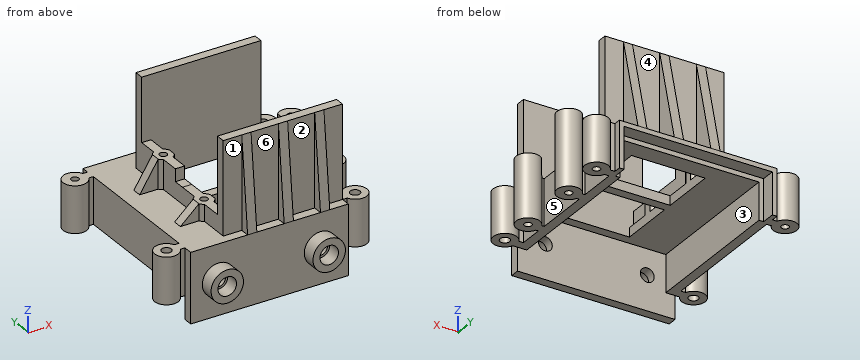
from build123d import *

# Parameters (mm, degrees)
ESQUISSE1_W              = 34
ESQUISSE1_H              = 15
BOSS_EXTRU_1_DEPTH       = 2
ESQUISSE2_R              = 1.5
ENL_V_MAT_EXTRU_1_DEPTH  = 2
BOSS_EXTRU_2_DEPTH       = 35
ENL_V_MAT_EXTRU_2_DEPTH  = 3
ESQUISSE5_R              = 3.5
ESQUISSE5_R_2            = 2
BOSS_EXTRU_3_DEPTH       = 3
ENL_V_START              = -2
ESQUISSE6_W              = 14
ESQUISSE6_H              = 12
ENL_V_MAT_EXTRU_3_DEPTH  = 2
ESQUISSE7_W              = 14
ESQUISSE7_H              = 12
ENL_V_MAT_EXTRU_4_DEPTH  = 2
ESQUISSE8_W              = 3
ESQUISSE8_H              = 12
ENL_V_MAT_EXTRU_5_DEPTH  = 2
BOSS_EXTRU_4_START       = -2
ESQUISSE9_W              = 1.1
ESQUISSE9_H              = 12
BOSS_EXTRU_4_DEPTH       = 2
ESQUISSE10_R             = 0.8
BOSS_EXTRU_5_DEPTH       = 6.285817
ESQUISSE11_R             = 0.8
BOSS_EXTRU_6_DEPTH       = 3.585817
ESQUISSE21_W             = 4
ESQUISSE21_H             = 2
BOSS_EXTRU_12_DEPTH      = 6.285817
ENL_V_MAT_EXTRU_9_DEPTH  = 2
ESQUISSE23_W             = 4
ESQUISSE23_H             = 2
BOSS_EXTRU_13_DEPTH      = 3.585817
ENL_V_MAT_EXTRU_10_DEPTH = 2
ESQUISSE25_W             = 2
ESQUISSE25_H             = 4.092832792
ESQUISSE25_H_2           = 4.443065592
BOSS_EXTRU_14_DEPTH      = 3.585817
ESQUISSE27_W             = 2
ESQUISSE27_H             = 4.092832792
ESQUISSE27_H_2           = 4
BOSS_EXTRU_15_DEPTH      = 6.285817
BOSS_EXTRU_17_START      = -10
ESQUISSE31_R             = 1.05
BOSS_EXTRU_17_DEPTH      = 10
BOSS_EXTRU_18_START      = -10
ESQUISSE33_R             = 0.8
BOSS_EXTRU_18_DEPTH      = 10
ESQUISSE34_R             = 0.8
BOSS_EXTRU_19_DEPTH      = 16.290743
ESQUISSE35_R             = 0.8
BOSS_EXTRU_20_DEPTH      = 13.590743
BOSS_EXTRU_21_DEPTH      = 20
ENL_V_START_2            = -17.727203
ENL_V_MAT_EXTRU_14_DEPTH = 17.727203
BOSS_EXTRU_23_START      = -2
ESQUISSE39_W             = 3.585817331
ESQUISSE39_H             = 2.443065592
BOSS_EXTRU_23_DEPTH      = 2
ENL_V_START_3            = -6.290743
ESQUISSE40_W             = 1.637082072
ESQUISSE40_H             = 4.811547665
ENL_V_MAT_EXTRU_15_DEPTH = 6.290743
ENL_V_START_4            = -3.590743
ESQUISSE41_W             = 1.862657742
ESQUISSE41_H             = 4.792301475
ENL_V_MAT_EXTRU_16_DEPTH = 3.590743
BOSS_EXTRU_24_DEPTH      = 20
ENL_V_MAT_EXTRU_17_DEPTH = 17.727203


with BuildPart() as part:
    # Esquisse1 → Boss.-Extru.1 (new body)
    with BuildSketch(Plane(origin=(0, 0, 0), x_dir=(1, 0, 0), z_dir=(0, 1, 0))):
        with Locations((17, 7.5)):
            Rectangle(ESQUISSE1_W, ESQUISSE1_H)
    extrude(amount=BOSS_EXTRU_1_DEPTH)

    # Esquisse2 → Enl_v. mat.-Extru.1 (cut)
    with BuildSketch(Plane(origin=(0, 2, 0), x_dir=(1, 0, 0), z_dir=(0, 1, 0))):
        with Locations((6, 7.5)):
            Circle(ESQUISSE2_R)
        with Locations((28, 7.5)):
            Circle(ESQUISSE2_R)
    extrude(amount=-ENL_V_MAT_EXTRU_1_DEPTH, mode=Mode.SUBTRACT)

    # Esquisse3 → Boss.-Extru.2 (add)
    with BuildSketch(Plane(origin=(0, 2, 0), x_dir=(1, 0, 0), z_dir=(0, 1, 0))):
        Polygon((0, 10), (2, 10), (2, 2), (32, 2), (32, 10), (34, 10), (34, 0), (0, 0), align=None)
    extrude(amount=BOSS_EXTRU_2_DEPTH)

    # Esquisse4 → Enl_v. mat.-Extru.2 (cut)
    with BuildSketch(Plane(origin=(0, 37, 0), x_dir=(1, 0, 0), z_dir=(0, 1, 0))):
        Polygon((2, 10), (1, 10), (1, 1), (33, 1), (33, 10), (32, 10), (32, 2), (2, 2), align=None)
    extrude(amount=-ENL_V_MAT_EXTRU_2_DEPTH, mode=Mode.SUBTRACT)

    # Esquisse5 → Boss.-Extru.3 (add)
    with BuildSketch(Plane.XZ):
        with Locations((6, -7.5)):
            Circle(ESQUISSE5_R)
        with Locations((6, -7.5)):
            Circle(ESQUISSE5_R_2, mode=Mode.SUBTRACT)
        with Locations((28, -7.5)):
            Circle(ESQUISSE5_R)
        with Locations((28, -7.5)):
            Circle(ESQUISSE5_R_2, mode=Mode.SUBTRACT)
    extrude(amount=BOSS_EXTRU_3_DEPTH)

    # Esquisse6 → Enl_v. mat.-Extru.3 (cut)
    with BuildSketch(Plane(origin=(0, 0, -2), x_dir=(-1, 0, 0), z_dir=(0, 0, -1)).offset(ENL_V_START)):
        with Locations((-17, 24)):
            Rectangle(ESQUISSE6_W, ESQUISSE6_H)
    extrude(amount=ENL_V_MAT_EXTRU_3_DEPTH, mode=Mode.SUBTRACT)

    # Esquisse7 → Enl_v. mat.-Extru.4 (cut)
    with BuildSketch(Plane(origin=(0, 0, -2), x_dir=(-1, 0, 0), z_dir=(0, 0, -1)).offset(ENL_V_START)):
        with Locations((-17, 10)):
            Rectangle(ESQUISSE7_W, ESQUISSE7_H)
    extrude(amount=ENL_V_MAT_EXTRU_4_DEPTH, mode=Mode.SUBTRACT)

    # Esquisse8 → Enl_v. mat.-Extru.5 (cut)
    with BuildSketch(Plane.XY.offset(ENL_V_START)):
        with Locations((25.5, 10)):
            Rectangle(ESQUISSE8_W, ESQUISSE8_H)
        with Locations((25.5, 24)):
            Rectangle(ESQUISSE8_W, ESQUISSE8_H)
    extrude(amount=ENL_V_MAT_EXTRU_5_DEPTH, mode=Mode.SUBTRACT)

    # Esquisse9 → Boss.-Extru.4 (add)
    with BuildSketch(Plane.XY.offset(BOSS_EXTRU_4_START)):
        with Locations((10.55, 24)):
            Rectangle(ESQUISSE9_W, ESQUISSE9_H)
        with Locations((10.55, 10)):
            Rectangle(ESQUISSE9_W, ESQUISSE9_H)
    extrude(amount=BOSS_EXTRU_4_DEPTH)

    # Esquisse10 → Boss.-Extru.5 (add)
    with BuildSketch(Plane.XY):
        with BuildLine():
            Line((11.1, 24.988338073), (11.1, 23.361894727))
            ThreePointArc((11.1, 23.361894727), (7.27279708, 24.1751164), (11.1, 24.988338073))
        make_face()
        with Locations((9.27279708, 24.1751164)):
            Circle(ESQUISSE10_R, mode=Mode.SUBTRACT)
    extrude(amount=BOSS_EXTRU_5_DEPTH)

    # Esquisse11 → Boss.-Extru.6 (add)
    with BuildSketch(Plane.XY):
        with BuildLine():
            Line((11.1, 10.988338073), (11.1, 9.361894727))
            ThreePointArc((11.1, 9.361894727), (7.27279708, 10.1751164), (11.1, 10.988338073))
        make_face()
        with Locations((9.27279708, 10.1751164)):
            Circle(ESQUISSE11_R, mode=Mode.SUBTRACT)
    extrude(amount=BOSS_EXTRU_6_DEPTH)

    # Esquisse21 → Boss.-Extru.12 (add)
    with BuildSketch(Plane.XY):
        with Locations((5.540746272, 24.1751164)):
            Rectangle(ESQUISSE21_W, ESQUISSE21_H)
    extrude(amount=BOSS_EXTRU_12_DEPTH)

    # Esquisse22 → Enl_v. mat.-Extru.9 (cut)
    with BuildSketch(Plane(origin=(0, 25.1751164, 0), x_dir=(1, 0, 0), z_dir=(0, 1, 0))):
        Polygon((3.540746272, 0), (7.540746272, -6.285817331), (3.540746272, -6.285817331), align=None)
    extrude(amount=-ENL_V_MAT_EXTRU_9_DEPTH, mode=Mode.SUBTRACT)

    # Esquisse23 → Boss.-Extru.13 (add)
    with BuildSketch(Plane.XY):
        with Locations((5.540746272, 10.1751164)):
            Rectangle(ESQUISSE23_W, ESQUISSE23_H)
    extrude(amount=BOSS_EXTRU_13_DEPTH)

    # Esquisse24 → Enl_v. mat.-Extru.10 (cut)
    with BuildSketch(Plane.XZ.offset(-9.1751164)):
        Polygon((7.540746272, 3.585817331), (3.540746272, 0), (3.540746272, 3.585817331), align=None)
    extrude(amount=-ENL_V_MAT_EXTRU_10_DEPTH, mode=Mode.SUBTRACT)

    # Esquisse25 → Boss.-Extru.14 (add)
    with BuildSketch(Plane.XY):
        with Locations((9.27279708, 13.953583604)):
            Rectangle(ESQUISSE25_W, ESQUISSE25_H)
        with Locations((9.27279708, 6.221532796)):
            Rectangle(ESQUISSE25_W, ESQUISSE25_H_2)
    extrude(amount=BOSS_EXTRU_14_DEPTH)

    # Esquisse27 → Boss.-Extru.15 (add)
    with BuildSketch(Plane.XY):
        with Locations((9.27279708, 27.953583604)):
            Rectangle(ESQUISSE27_W, ESQUISSE27_H)
        with Locations((9.27279708, 20.443065592)):
            Rectangle(ESQUISSE27_W, ESQUISSE27_H_2)
    extrude(amount=BOSS_EXTRU_15_DEPTH)

    # Esquisse31 → Boss.-Extru.17 (add)
    with BuildSketch(Plane.XY.offset(BOSS_EXTRU_17_START)):
        with BuildLine():
            Line((-1, 4), (0, 4))
            Line((0, 4), (0, 2))
            Line((0, 2), (-1, 2))
            ThreePointArc((-1, 2), (-5.895740821, 3), (-1, 4))
        make_face()
        with Locations((-3.345740821, 3)):
            Circle(ESQUISSE31_R, mode=Mode.SUBTRACT)
        with BuildLine():
            Line((34, 4), (34, 2))
            Line((34, 2), (35, 2))
            ThreePointArc((35, 2), (39.895740821, 3), (35, 4))
            Line((35, 4), (34, 4))
        make_face()
        with Locations((37.345740821, 3)):
            Circle(ESQUISSE31_R, mode=Mode.SUBTRACT)
    extrude(amount=BOSS_EXTRU_17_DEPTH)

    # Esquisse33 → Boss.-Extru.18 (add)
    with BuildSketch(Plane.XY.offset(BOSS_EXTRU_18_START)):
        with BuildLine():
            Line((35, 33.45), (34, 33.45))
            Line((34, 33.45), (34, 35.45))
            Line((34, 35.45), (35, 35.45))
            ThreePointArc((35, 35.45), (39.895740821, 34.45), (35, 33.45))
        make_face()
        with Locations((37.345740821, 34.45)):
            Circle(ESQUISSE33_R, mode=Mode.SUBTRACT)
        with BuildLine():
            Line((0, 33.45), (0, 35.45))
            Line((0, 35.45), (-1, 35.45))
            ThreePointArc((-1, 35.45), (-5.895740821, 34.45), (-1, 33.45))
            Line((-1, 33.45), (0, 33.45))
        make_face()
        with Locations((-3.345740821, 34.45)):
            Circle(ESQUISSE33_R, mode=Mode.SUBTRACT)
    extrude(amount=BOSS_EXTRU_18_DEPTH)

    # Esquisse34 → Boss.-Extru.19 (add)
    with BuildSketch(Plane(origin=(0, 0, -10), x_dir=(-1, 0, 0), z_dir=(0, 0, -1))):
        with BuildLine():
            Line((-34.527056259, 25.1751164), (-34, 25.1751164))
            Line((-34, 25.1751164), (-34, 23.1751164))
            Line((-34, 23.1751164), (-34.527056259, 23.1751164))
            ThreePointArc((-34.527056259, 23.1751164), (-39.42279708, 24.1751164), (-34.527056259, 25.1751164))
        make_face()
        with Locations((-36.87279708, 24.1751164)):
            Circle(ESQUISSE34_R, mode=Mode.SUBTRACT)
    extrude(amount=-BOSS_EXTRU_19_DEPTH)

    # Esquisse35 → Boss.-Extru.20 (add)
    with BuildSketch(Plane(origin=(0, 0, -10), x_dir=(-1, 0, 0), z_dir=(0, 0, -1))):
        with BuildLine():
            Line((-34.527056259, 11.1751164), (-34, 11.1751164))
            Line((-34, 11.1751164), (-34, 9.1751164))
            Line((-34, 9.1751164), (-34.527056259, 9.1751164))
            ThreePointArc((-34.527056259, 9.1751164), (-39.42279708, 10.1751164), (-34.527056259, 11.1751164))
        make_face()
        with Locations((-36.87279708, 10.1751164)):
            Circle(ESQUISSE35_R, mode=Mode.SUBTRACT)
    extrude(amount=-BOSS_EXTRU_20_DEPTH)

    # Esquisse36 → Boss.-Extru.21 (add)
    with BuildSketch(Plane.XY):
        Polygon((8.27279708, 30), (34, 30), (34, 32), (30, 32), (30, 37), (28.05279708, 37), (28.05279708, 32), (22.16279708, 32), (22.16279708, 37), (20.16279708, 37), (20.16279708, 32), (14.27279708, 32), (14.27279708, 37), (12.27279708, 37), (12.27279708, 32), (8.27279708, 32), align=None)
    extrude(amount=BOSS_EXTRU_21_DEPTH)

    # Esquisse37 → Enl_v. mat.-Extru.14 (cut)
    with BuildSketch(Plane(origin=(30, 0, 0), x_dir=(0, 0, -1), z_dir=(1, 0, 0)).offset(ENL_V_START_2)):
        Polygon((-20, 32), (0, 37), (-20, 37), align=None)
    extrude(amount=ENL_V_MAT_EXTRU_14_DEPTH, mode=Mode.SUBTRACT)

    # Esquisse39 → Boss.-Extru.23 (add)
    with BuildSketch(Plane.ZY.offset(-8.27279708).offset(BOSS_EXTRU_23_START)):
        with Locations((1.792908666, 17.221532796)):
            Rectangle(ESQUISSE39_W, ESQUISSE39_H)
    extrude(amount=BOSS_EXTRU_23_DEPTH)

    # Esquisse40 → Enl_v. mat.-Extru.15 (cut)
    with BuildSketch(Plane.XY.offset(6.290743087).offset(ENL_V_START_3)):
        with Locations((34.181130377, 24.126818711)):
            Rectangle(ESQUISSE40_W, ESQUISSE40_H)
    extrude(amount=ENL_V_MAT_EXTRU_15_DEPTH, mode=Mode.SUBTRACT)

    # Esquisse41 → Enl_v. mat.-Extru.16 (cut)
    with BuildSketch(Plane.XY.offset(3.590743087).offset(ENL_V_START_4)):
        with Locations((34.068342542, 10.376328553)):
            Rectangle(ESQUISSE41_W, ESQUISSE41_H)
    extrude(amount=ENL_V_MAT_EXTRU_16_DEPTH, mode=Mode.SUBTRACT)

    # Esquisse43 → Boss.-Extru.24 (add)
    with BuildSketch(Plane.XY):
        Polygon((14.27279708, 2), (20.16279708, 2), (20.16279708, 0), (22.16279708, 0), (22.16279708, 2), (28, 2), (28, 0), (30, 0), (30, 2), (34, 2), (34, 4), (8.27279708, 4), (8.27279708, 2), (12.27279708, 2), (12.27279708, 0), (14.27279708, 0), align=None)
    extrude(amount=BOSS_EXTRU_24_DEPTH)

    # Esquisse44 → Enl_v. mat.-Extru.17 (cut)
    with BuildSketch(Plane.ZY.offset(-12.27279708).offset(ENL_V_START_2)):
        Polygon((20, 2), (0, 0), (20, 0), align=None)
    extrude(amount=ENL_V_MAT_EXTRU_17_DEPTH, mode=Mode.SUBTRACT)


solid = part.part
Model file for the job. Use its own axes, mm. Face numbers are marked on the shaded views. A direction names the side the tool comes from. Round coordinates to 2 decimals unless told otherwise and drop trailing zeros. Loops run counter-clockwise (first coordinate to the right, second up) from the corner with the lowest first, then second, coordinate; pieces in that order, holes last. Notation, with made-up numbers: M -5.5,22 L 45.5,22 A11 ccw 45.5,34 Z; hole C 1.25,88 d5. An arc over 180 degrees is marked long. One line per question, with ' | ' between items.
1) 3-axis set-ups, long thin cutter, end or side, ignore diameter. For the marked faces 3, 4, 5 and 6: which of +Z, -Z, +X, -X, +Y, -Y reach the whole face in a straight line?
Solved:
face 3: -Z, +Y | face 4: +Z, +Y | face 5: +Z, -Z | face 6: +Z, -Y
2) Mould opens along X. For the marked faces 1 and 2 say: +X half, -X half, draft (parallel to the pull), parting line (faces both ways), or undercut.
Solved:
face 1: draft | face 2: undercut
3) Band-saw the part on D-D (y = 17). Give the cut face in (x, z), then the cut area to 3 significant figures.
Solved:
outline: M 0,-10 L 2,-10 L 2,-2 L 32,-2 L 32,-10 L 34,-10 L 34,0 L 10.27,0 L 10.27,3.59 L 8.27,3.59 L 8.27,0 L 0,0 Z | area: 107 mm²
4) Band-saw the part on A-A (x = 21.5). Give the cut face in (y, z), then the cut area to 3 significant figures.
Solved:
outline: M 0,-15 L 2,-15 L 2,-2 L 4,-2 L 4,20 L 2,20 L 0,0 Z; M 16,-2 L 18,-2 L 18,0 L 16,0 Z; M 30,-2 L 34,-2 L 34,-1 L 37,-1 L 37,0 L 32,20 L 30,20 Z | area: 199 mm²
5) Flat gauge pins, fed straight in: pin 1 (6.5 mm diameter, centred on y = 28, z = 9.5, fed in from -X); pin 2 (12 mm diameter, centred on y = 21.5, z = 0, fed in from +X); pin 3 (3 mm diameter, centred on y = 18, z = 3, fed in from +X). Where does each tip first touch, or does it go through?
Solved:
pin 1: stops at x = 8.27 | pin 2: stops at x = 39.42 | pin 3: stops at x = 10.27
6) Drill centre lines: line 1 along Y through (x, z) = (25, -0.5); line 2 along X through (y, z) = (1.35, -7.5); line 3 along X through (y, z) = (1, -1). Where is each one in solid material? Low to high.
Solved:
line 1: y = 0 to 4, 16 to 18, 30 to 37 | line 2: x = -5.29 to -1.4, 0 to 4.5, 7.5 to 26.5, 29.5 to 34, 35.4 to 39.29 | line 3: x = -4.93 to -1.76, 0 to 34, 35.76 to 38.93
7) Band-saw the part on B-B (y = 3). Give the cut face in (x, z).
Solved:
outline: M -5.9,-10 L -4.4,-10 L -4.4,0 L -5.9,0 Z; M -2.3,-10 L 2,-10 L 2,-2 L 32,-2 L 32,-10 L 36.3,-10 L 36.3,0 L 34,0 L 34,20 L 8.27,20 L 8.27,0 L -2.3,0 Z; M 38.4,-10 L 39.9,-10 L 39.9,0 L 38.4,0 Z
